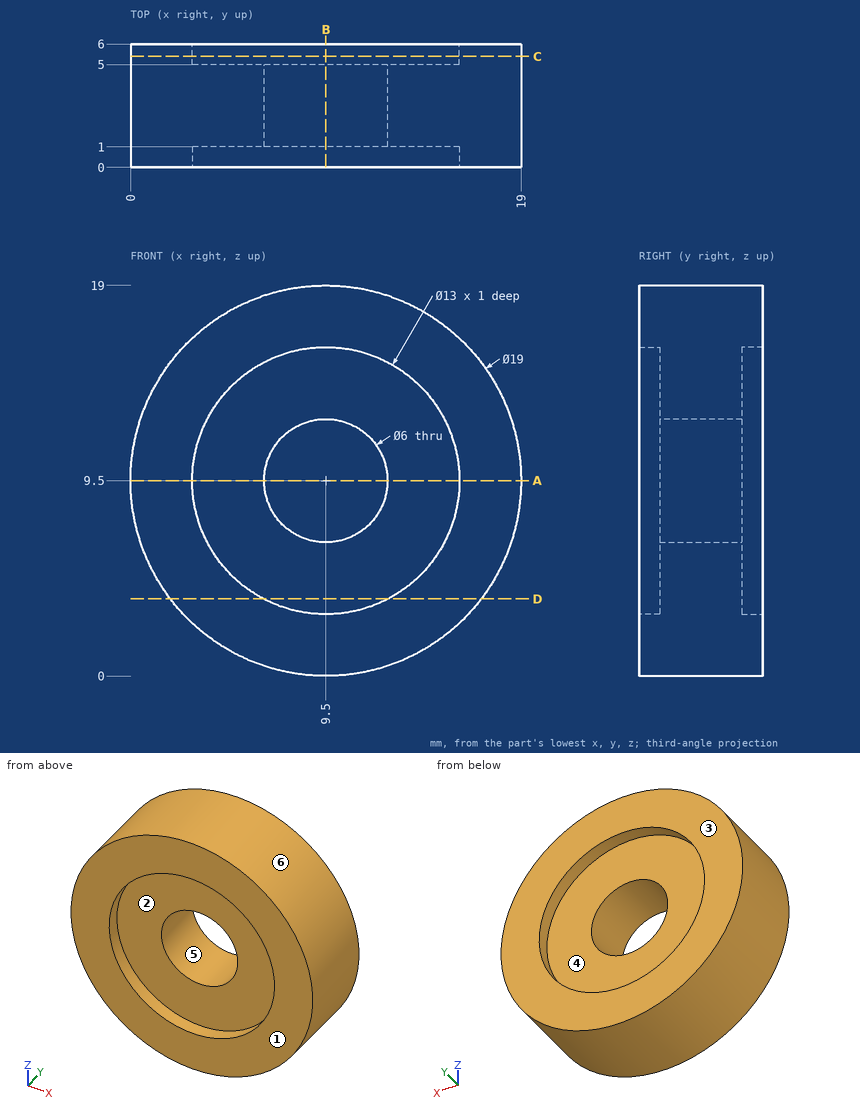
Job drawing, mm, ordinate dimensions from the low corner. One solid piece. A direction names the side the tool comes from. Round coordinates to 2 decimals unless told otherwise and drop trailing zeros. Loops run counter-clockwise (first coordinate to the right, second up) from the corner with the lowest first, then second, coordinate; pieces in that order, holes last. Notation, with made-up numbers: M -18,84 L 26,84 A18 ccw 26,111 Z; hole C 15,12.25 d8. An arc over 180 degrees is marked long. One line per question, with ' | ' between items. Start each with the question number.
Item 1: Cut at B-B, the plane x = 9.5. Write the cut outline in (y, z).
Item 2: Wall check: line 1 (X direction, y = 0.65, z = 9.5); line 2 (X direction, y = 2.5, z = 9.5); line 3 (Z direction, x = 11, y = 1.35). Give the ranges that are in metal, low to high.
Item 3: Two-plate mould, pull along Z, no slides. Class the marked faces 3, 4, 5 and 6: pulls with the +Z half, pulls with the -Z half, needs draft (parallel to the pull), parting line crosses it, or undercut.
Item 4: Cut at D-D, the plane z = 3.75. Write the cut outline in (x, y).
Item 5: Cut at C-C, the plane y = 5.4. Write the cut outline in (x, z).
Item 6: Pin check, flat tips, straight feed: pin 1 Ø7 at (x, z) = (9.5, 9.5) entering from +Y; pin 2 Ø1.5 at (y, z) = (4.5, 15) entering from -X. Stop position of each tip, or through.
Item 7: Cut at A-A, the plane z = 9.5. Write the cut outline in (x, y).
Item 8: Which spindle directions (+Z, -Z, +X, -X, +Y, -Y) get a long thin tool onto all of the face, cutting with end or side? Do the marked faces 1 and 2. Say none if no direction does.
Responses:
1) outline: M 0,0 L 6,0 L 6,3 L 5,3 L 5,6.5 L 1,6.5 L 1,3 L 0,3 Z; M 0,16 L 1,16 L 1,12.5 L 5,12.5 L 5,16 L 6,16 L 6,19 L 0,19 Z
2) line 1: x = 0 to 3, 16 to 19 | line 2: x = 0 to 6.5, 12.5 to 19 | line 3: z = 0.12 to 6.9, 12.1 to 18.88
3) face 3: needs draft | face 4: undercut | face 5: undercut | face 6: parting line crosses it
4) outline: M 1.94,0 L 6.47,0 L 6.47,1 L 12.53,1 L 12.53,0 L 17.06,0 L 17.06,6 L 12.53,6 L 12.53,5 L 6.47,5 L 6.47,6 L 1.94,6 Z
5) outline: C 9.5,9.5 d19; hole C 9.5,9.5 d13
6) pin 1: stops at y = 5 | pin 2: stops at x = 1.27
7) outline: M 0,0 L 3,0 L 3,1 L 6.5,1 L 6.5,5 L 3,5 L 3,6 L 0,6 Z; M 12.5,1 L 16,1 L 16,0 L 19,0 L 19,6 L 16,6 L 16,5 L 12.5,5 Z
8) face 1: +Z, -Z, +X, -X, -Y | face 2: -Y
